Can you work these out from the drawing? Everything is in mm from the part's minimum corner. Give positions to 0.01 mm unless a question says otherwise; leave off trailing zeros. Order: outer loops, then holes, each group sorted by start corner. A loop starts at its lowest first (then second) coordinate and runs counter-clockwise, first axis right, second up. Notation, with made-up numbers: M 16.5,5 L 37.5,5 A17 ccw 37.5,20 Z; hole C 58.25,54.25 d4. An arc over 180 degrees is marked long. Answer as a JSON object with one key per item and string values.
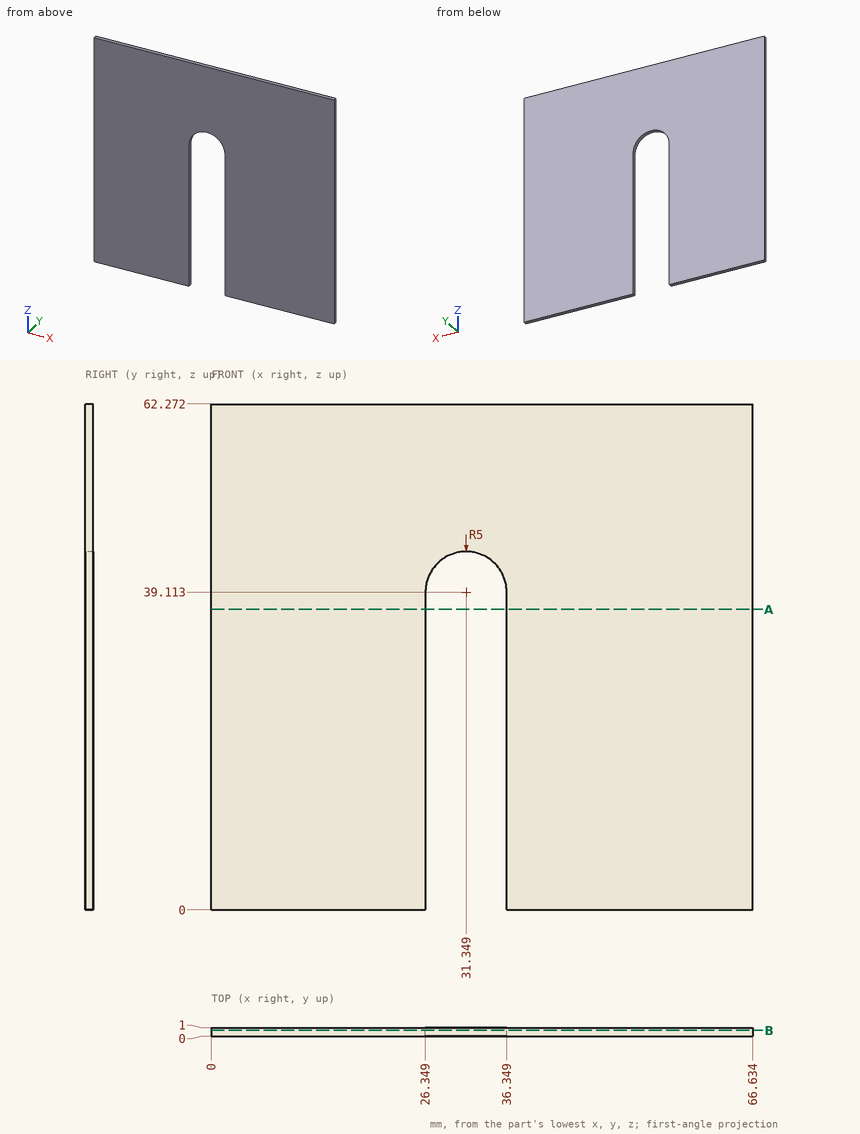
1) I want a section at B-B on y = 0.7. Write out the boundary of the cut face in (x, z).
Results found:
{"outline": "M 0,0 L 26.35,0 L 26.35,39.11 A5 cw 36.35,39.11 L 36.35,0 L 66.63,0 L 66.63,62.27 L 0,62.27 Z"}
2) I need wall thicknesses on L1, parallel to X at y = 0.7, z = 13.5; L2, parallel to Z at x = 31.5, y = 0.9; L3, parallel to X at y = 0.5, z = 42 (1 decimal). Which ranges of each line are inside material? Lowest first, please.
Results found:
{"L1": "x = 0 to 26.35, 36.35 to 66.63", "L2": "z = 44.11 to 62.27", "L3": "x = 0 to 27.3, 35.4 to 66.6"}
3) I want a section at A-A on z = 37. Write out the boundary of the cut face in (x, y).
Results found:
{"outline": "M 0,0 L 26.35,0 L 26.35,1 L 0,1 Z; M 36.35,0 L 66.63,0 L 66.63,1 L 36.35,1 Z"}
